```python
from build123d import *

# Parameters (mm, degrees)
BOSS_EXTRUDE1_DEPTH = 27.5
SKETCH3_W           = 15
SKETCH3_H           = 40
BOSS_EXTRUDE2_DEPTH = 8
SKETCH4_R           = 1.25
CUT_EXTRUDE1_DEPTH  = 70.371250359
CUT_EXTRUDE2_START  = -6
SKETCH4_3_R         = 2
SKETCH4_3_R_2       = 1.25
CUT_EXTRUDE2_DEPTH  = 2
SKETCH5_R           = 1.5
CUT_EXTRUDE3_DEPTH  = 84.963392862
SKETCH5_3_R         = 3
SKETCH5_3_R_2       = 1.5
CUT_EXTRUDE4_DEPTH  = 3
FILLET1_R           = 4


with BuildPart() as part:
    # Sketch1 → Boss-Extrude1 (new body)
    with BuildSketch(Plane.XY):
        with BuildLine():
            Line((-27.263565268, -0.826290167), (-27.263565268, 39.032085652))
            ThreePointArc((-27.263565268, 39.032085652), (-23.226265639, 43.618644017), (-17.274109595, 45))
            Line((-17.274109595, 45), (15.736434732, 45))
            Line((15.736434732, 45), (15.736434732, -0.826290167))
            Line((15.736434732, -0.826290167), (23.736434732, -0.826290167))
            Line((23.736434732, -0.826290167), (23.736434732, 53))
            Line((23.736434732, 53), (-16.992356062, 53))
            ThreePointArc((-16.992356062, 53), (-28.288998955, 49.870920305), (-35.263565268, 40.449630311))
            Line((-35.263565268, 40.449630311), (-35.263565268, -0.826290167))
            Line((-35.263565268, -0.826290167), (-27.263565268, -0.826290167))
        make_face()
    extrude(amount=BOSS_EXTRUDE1_DEPTH)

    # Sketch3 → Boss-Extrude2 (add)
    with BuildSketch(Plane(origin=(0, 0, 0), x_dir=(-1, 0, 0), z_dir=(0, 0, -1))):
        with Locations((-16.236434732, 33)):
            Rectangle(SKETCH3_W, SKETCH3_H)
    extrude(amount=BOSS_EXTRUDE2_DEPTH)

    # Sketch4 → Cut-Extrude1 (cut, through all)
    with BuildSketch(Plane.XY):
        with Locations((12.736434732, 42.5)):
            Circle(SKETCH4_R)
        with Locations((12.736434732, 15.5)):
            Circle(SKETCH4_R)
    extrude(amount=-CUT_EXTRUDE1_DEPTH, mode=Mode.SUBTRACT)

    # Sketch4<3> → Cut-Extrude2 (cut)
    # profile 1 of 2: a face of its own
    with BuildSketch(Plane.XY.offset(CUT_EXTRUDE2_START)):
        with Locations(Location((12.736434732, 42.5, 0), (0, 0, 180))):
            Circle(SKETCH4_3_R)
        with Locations((12.736434732, 42.5)):
            Circle(SKETCH4_3_R_2, mode=Mode.SUBTRACT)
    # profile 2 of 2: a face of its own
    with BuildSketch(Plane.XY.offset(CUT_EXTRUDE2_START)):
        with Locations(Location((12.736434732, 15.5, 0), (0, 0, 180))):
            Circle(SKETCH4_3_R)
        with Locations((12.736434732, 15.5)):
            Circle(SKETCH4_3_R_2, mode=Mode.SUBTRACT)
    extrude(amount=-CUT_EXTRUDE2_DEPTH, mode=Mode.SUBTRACT)

    # Sketch5 → Cut-Extrude3 (cut, through all)
    with BuildSketch(Plane(origin=(23.736434732, 0, 0), x_dir=(0, 0, -1), z_dir=(1, 0, 0))):
        with Locations((-22.5, 6.086854916)):
            Circle(SKETCH5_R)
        with Locations((-5, 6.086854916)):
            Circle(SKETCH5_R)
    extrude(amount=-CUT_EXTRUDE3_DEPTH, mode=Mode.SUBTRACT)

    # Sketch5<3> → Cut-Extrude4 (cut)
    # profile 1 of 2: a face of its own
    with BuildSketch(Plane(origin=(23.736434732, 0, 0), x_dir=(0, 0, -1), z_dir=(1, 0, 0))):
        with Locations((-22.5, 6.086854916)):
            Circle(SKETCH5_3_R)
        with Locations((-22.5, 6.086854916)):
            Circle(SKETCH5_3_R_2, mode=Mode.SUBTRACT)
    # profile 2 of 2: a face of its own
    with BuildSketch(Plane(origin=(23.736434732, 0, 0), x_dir=(0, 0, -1), z_dir=(1, 0, 0))):
        with Locations((-5, 6.086854916)):
            Circle(SKETCH5_3_R)
        with Locations((-5, 6.086854916)):
            Circle(SKETCH5_3_R_2, mode=Mode.SUBTRACT)
    cut_extrude4 = extrude(amount=-CUT_EXTRUDE4_DEPTH, mode=Mode.SUBTRACT)

    # Mirror1: Cut-Extrude4 across plane
    add(cut_extrude4.mirror(Plane(origin=(-5.763565268, 0, 0), x_dir=(0, 0, 1), z_dir=(1, 0, 0))), mode=Mode.SUBTRACT)

    # Fillet1
    fillet1_edges = [part.edges().sort_by_distance(p)[0] for p in [
        (23.736434732, 53, 9.75),
    ]]
    fillet(fillet1_edges, radius=FILLET1_R)


solid = part.part
```
CAD build for the part. Positions are in the model's coordinates, mm. A direction names the side the tool comes from. Coordinates: 2 decimals unless noted, no trailing zeros. Write each loop counter-clockwise with the first axis right and the second up, starting at its lowest first coordinate (ties: lowest second). Pieces come first, ordered by that corner, then holes.
(1) Drill centre lines: probe 1 along X at (y, z) = (6.5, 6.5); probe 2 along X at (y, z) = (42.5, -7.05); probe 3 along Y at (x, z) = (18.95, 5). Where is each one in solid material? Low to high.
(2) Cut at D-D, the plane z = 15. List the corners of the cut face in (x, y).
(3) 3-axis set-ups, long thin cutter, end or side, ignore diameter. For faces 1 (the face through (-32.264, 4.8, 3.7)), 2 (the face through (20, 6, 0)), 3 (the face through (22.257, 6.219, 25.497)), 4 (the face through (13, 44, -6)): which of +Z, -Z, +X, -X, +Y, -Y reach the whole face in a straight line?
(4) Cut at A-A, the plane y = 15.5. List the corners of the cut face in (x, z).
(5) Two-plate mould, pull along Z, no slides. Class faces 5 (the face through (-27.264, 19, 14)), 6 (the face through (12, 29, 0)), 7 (the face through (22.26, 6.99, 2.14)), 8 (the face through (18.271, 4.623, 5.325)): +Z half, -Z half, draft (parallel to the pull), parting line (faces both ways), or undercut.
(6) Flat gauge pins, fed straight in: pin 1 (4 mm diameter, centred on y = 6.09, z = 5, fed in from -X); pin 2 (3 mm diameter, centred on y = 7, z = 22, fed in from +X); pin 3 (4 mm diameter, centred on x = 12.74, y = 42.5, fed in from +Z). Where does each tip first touch, or does it go through?
(7) Cut at C-C, the plane y = 23. List the corners of the cut face in (x, z).
(8) Cut at B-B, the plane z = 5. List the corners of the cut face in (x, y), and give its area (3 significant figures).
Geometry says:
1. probe 1: x = -32.26 to -27.26, 15.74 to 20.74
1. probe 2: x = 8.74 to 10.74, 14.74 to 23.74
1. probe 3: y = -0.83 to 4.59, 7.59 to 53
2. outline: (-35.26, -0.83) - (-27.26, -0.83) - (-27.26, 39.03) arc R10 cw to (-17.27, 45) - (15.74, 45) - (15.74, -0.83) - (23.74, -0.83) - (23.74, 49) arc R4 ccw to (19.74, 53) - (-16.99, 53) arc R18 ccw to (-35.26, 40.45) - close
3. face 1: -X
3. face 2: -Z, +X, -X, -Y
3. face 3: +X
3. face 4: -Z
4. outline: (-35.26, 0) - (-27.26, 0) - (-27.26, 27.5) - (-35.26, 27.5) - close; (8.74, -8) - (10.74, -8) - (10.74, -6) - (11.49, -6) - (11.49, 0) - (8.74, 0) - close; (13.99, -6) - (14.74, -6) - (14.74, -8) - (23.74, -8) - (23.74, 27.5) - (15.74, 27.5) - (15.74, 0) - (13.99, 0) - close
5. face 5: draft
5. face 6: +Z half
5. face 7: undercut
5. face 8: undercut
6. pin 1: stops at x = -32.26
6. pin 2: stops at x = 20.74
6. pin 3: stops at z = 0
7. outline: (-35.26, 0) - (-27.26, 0) - (-27.26, 27.5) - (-35.26, 27.5) - close; (8.74, -8) - (23.74, -8) - (23.74, 27.5) - (15.74, 27.5) - (15.74, 0) - (8.74, 0) - close
8. outline: (-35.26, -0.83) - (-27.26, -0.83) - (-27.26, 4.59) - (-32.26, 4.59) - (-32.26, 3.09) - (-35.26, 3.09) - close; (-35.26, 9.09) - (-32.26, 9.09) - (-32.26, 7.59) - (-27.26, 7.59) - (-27.26, 39.03) arc R10 cw to (-17.27, 45) - (15.74, 45) - (15.74, 7.59) - (20.74, 7.59) - (20.74, 9.09) - (23.74, 9.09) - (23.74, 49) arc R4 ccw to (19.74, 53) - (-16.99, 53) arc R18 ccw to (-35.26, 40.45) - close; (15.74, -0.83) - (23.74, -0.83) - (23.74, 3.09) - (20.74, 3.09) - (20.74, 4.59) - (15.74, 4.59) - close
8. area: 1,090 mm2
